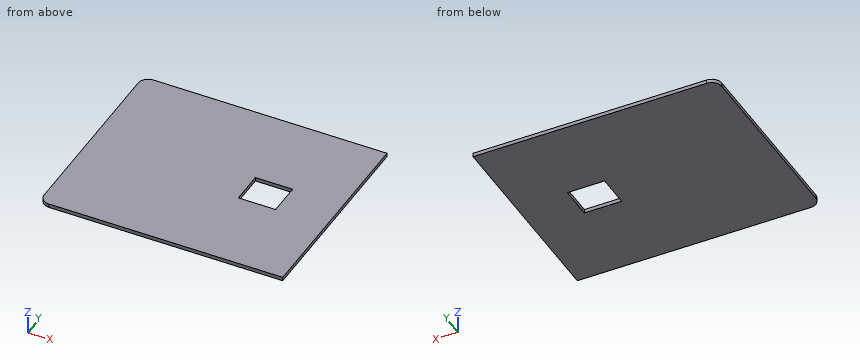
```python
from build123d import *

# Parameters (mm, degrees)
F1_DEPTH = 28.575
F3_DEPTH = 28.575


with BuildPart() as f1:
    # F0 (on Top) → F1 (new body)
    with BuildSketch(Plane.XY):
        with BuildLine():
            Line((914.4, -762), (914.4, 762))
            Line((914.4, 762), (-838.2, 762))
            ThreePointArc((-838.2, 762), (-892.081537, 739.681537), (-914.4, 685.8))
            Line((-914.4, 685.8), (-914.4, -685.8))
            ThreePointArc((-914.4, -685.8), (-892.081537, -739.681537), (-838.2, -762))
            Line((-838.2, -762), (914.4, -762))
        make_face()
    extrude(amount=F1_DEPTH)

    # F2 (on face) → F3 (cut)
    with BuildSketch(Plane.XY.offset(28.575)):
        Polygon((533.4, -124.587), (533.4, 0), (533.4, 124.587), (254, 124.587), (254, -124.587), align=None)
    extrude(amount=-F3_DEPTH, mode=Mode.SUBTRACT)


solid = f1.part
```
Read the model definition and answer for the solid it produces. Units are mm, in the model's axes. Give positions to 0.01 mm unless a question says otherwise; leave off trailing zeros. Order: outer loops, then holes, each group sorted by start corner. A loop starts at its lowest first (then second) coordinate and runs counter-clockwise, first axis right, second up. Notation, with made-up numbers: (-12, 40.25) -> (38, 40.25) arc R22 cw to (38, 73.25) -> close; hole circle Ø10 at (73.5, 17). An arc over 180 degrees is marked (long way). One line per item, written item: value. Start each with the question number.
(1) The part is cut by section B-B (y = -90.5). Determine the outline of the cut face in (x, z) (3 decimals), and give its area (3 significant figures).
(2) Straight lines are drawn through the part: L1, parallel to Y at x = 301, z = 13.75; L2, parallel to X at y = -10, z = 6.75; L3, parallel to X at y = -690.5, z = 10. For each, find the intervals that lie inside material, in ascending order.
(3) The part is cut by section C-C (x = 493). Determine the outline of the cut face in (y, z) (3 decimals), and give its area (3 significant figures).
(4) The part is cut by section A-A (z = 15). Determine the outline of the cut face in (x, y), and give its area (3 significant figures).
Taken from the geometry:
1. outline: (-914.4, 0) -> (254, 0) -> (254, 28.575) -> (-914.4, 28.575) -> close; (533.4, 0) -> (914.4, 0) -> (914.4, 28.575) -> (533.4, 28.575) -> close
1. area: 44,300 mm^2
2. L1: -762 to -124.59, 124.59 to 762
2. L2: -914.4 to 254, 533.4 to 914.4
2. L3: -914.25 to 914.4
3. outline: (-762, 0) -> (-124.587, 0) -> (-124.587, 28.575) -> (-762, 28.575) -> close; (124.587, 0) -> (762, 0) -> (762, 28.575) -> (124.587, 28.575) -> close
3. area: 36,400 mm^2
4. outline: (-914.4, -685.8) arc R76.2 ccw to (-838.2, -762) -> (914.4, -762) -> (914.4, 762) -> (-838.2, 762) arc R76.2 ccw to (-914.4, 685.8) -> close; hole (254, -124.59) -> (533.4, -124.59) -> (533.4, 124.59) -> (254, 124.59) -> close
4. area: 2,710,000 mm^2
